Design review of the part built by this model. Coordinates are the model's own, in mm. Give positions to 0.01 mm unless a question says otherwise; leave off trailing zeros. Order: outer loops, then holes, each group sorted by start corner. A loop starts at its lowest first (then second) coordinate and runs counter-clockwise, first axis right, second up.
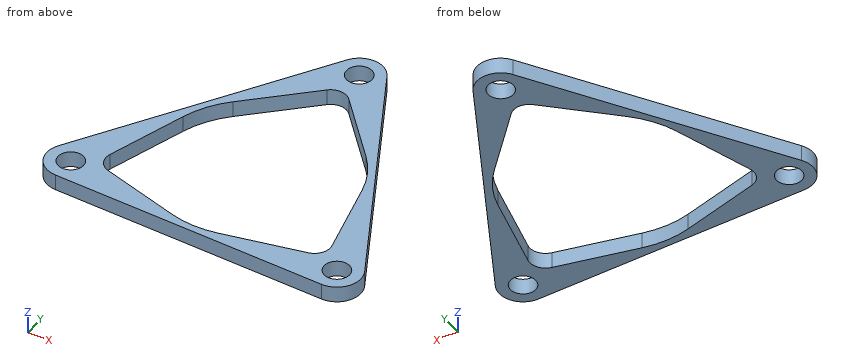
```python
from build123d import *

# Parameters (mm, degrees)
SKETCH1_R           = 3
SKETCH1_R_2         = 1.6
BOSS_EXTRUDE1_DEPTH = 2


with BuildPart() as part:
    # Sketch1 → Boss-Extrude1 (new body)
    # profile 1 of 4: a face of its own
    with BuildSketch(Plane.XY):
        with BuildLine():
            ThreePointArc((3.814909487, 19.983391167), (-0.020434351, 17.102037202), (-1.719890963, 21.588005352))
            Line((-1.719890963, 21.588005352), (-20.248379597, -7.681349081))
            ThreePointArc((-20.248379597, -7.681349081), (-16.87823531, -6.404609301), (-14.713579148, -9.285963266))
            ThreePointArc((-14.713579148, -9.285963266), (-15.635925335, -11.450069233), (-17.835815571, -12.283471941))
            Line((-17.835815571, -12.283471941), (16.776433238, -13.694936576))
            ThreePointArc((16.776433238, -13.694936576), (14.363869212, -9.092813716), (19.555706533, -9.304533411))
            Line((19.555706533, -9.304533411), (3.471946359, 21.376285657))
            ThreePointArc((3.471946359, 21.376285657), (3.727907136, 20.700639166), (3.814909487, 19.983391167))
        make_face()
        with BuildLine():
            Line((-8.306162696, 8.798730663), (-0.783837106, 15.899943621))
            ThreePointArc((-0.783837106, 15.899943621), (0.670573296, 16.443947091), (2.075859948, 15.783327064))
            Line((2.075859948, 15.783327064), (8.995004486, 8.093200498))
            ThreePointArc((8.995004486, 8.093200498), (10.716715384, 5.618007776), (11.773005623, 2.793982571))
            Line((11.773005623, 2.793982571), (14.161673647, -7.271148964))
            ThreePointArc((14.161673647, -7.271148964), (13.905589271, -8.802707055), (12.63083222, -9.689410982))
            Line((12.63083222, -9.689410982), (2.511414986, -11.836502641))
            ThreePointArc((2.511414986, -11.836502641), (-0.493020239, -12.089951656), (-3.466842927, -11.592713234))
            Line((-3.466842927, -11.592713234), (-13.377836541, -8.628794657))
            ThreePointArc((-13.377836541, -8.628794657), (-14.576162567, -7.641240036), (-14.706692168, -6.093916082))
            Line((-14.706692168, -6.093916082), (-11.506419472, 3.743302143))
            ThreePointArc((-11.506419472, 3.743302143), (-10.223695145, 6.47194388), (-8.306162696, 8.798730663))
        make_face(mode=Mode.SUBTRACT)
    # profile 2 of 4: a face of its own
    with BuildSketch(Plane.XY):
        with Locations((0.814909487, 19.983391167)):
            Circle(SKETCH1_R)
        with Locations((0.814909487, 19.983391167)):
            Circle(SKETCH1_R_2, mode=Mode.SUBTRACT)
    # profile 3 of 4: a face of its own
    with BuildSketch(Plane.XY):
        with Locations((16.898669661, -10.697427901)):
            Circle(SKETCH1_R)
        with Locations((16.898669661, -10.697427901)):
            Circle(SKETCH1_R_2, mode=Mode.SUBTRACT)
    # profile 4 of 4: a face of its own
    with BuildSketch(Plane.XY):
        with Locations((-17.713579148, -9.285963266)):
            Circle(SKETCH1_R)
        with Locations((-17.713579148, -9.285963266)):
            Circle(SKETCH1_R_2, mode=Mode.SUBTRACT)
    extrude(amount=BOSS_EXTRUDE1_DEPTH)


solid = part.part
```
1. Take a section at C-C (z = 1.1). State the section outline as (x, y) points (1 decimal), then the cut area to 3 significant figures.
Recorded:
outline: (-20.2, -7.7) arc R3 ccw to (-17.8, -12.3) - (16.8, -13.7) arc R3 ccw to (19.6, -9.3) - (3.5, 21.4) arc R3 ccw to (-1.7, 21.6) - close; hole circle Ø3.2 at (-17.7, -9.3); hole (-14.7, -6.1) arc R2 ccw to (-13.4, -8.6) - (-3.5, -11.6) arc R12.1 ccw to (2.5, -11.8) - (12.6, -9.7) arc R2 ccw to (14.2, -7.3) - (11.8, 2.8) arc R12.1 ccw to (9, 8.1) - (2.1, 15.8) arc R2 ccw to (-0.8, 15.9) - (-8.3, 8.8) arc R12.1 ccw to (-11.5, 3.7) - close; hole circle Ø3.2 at (0.8, 20); hole circle Ø3.2 at (16.9, -10.7)
area: 279 mm2
2. For pin 1 (1 mm diameter, centred on x = -3, z = 0.5, fed in from -Y), flat-tipped, find the tip position at first contact; note if it passes through.
Recorded:
pin 1: stops at y = -12.91
3. Take a section at D-D (y = 17). State the section outline as (x, z) points.
Recorded:
outline: (-4.62, 0) - (5.77, 0) - (5.77, 2) - (-4.62, 2) - close
4. For line 1 along Y through (x, z) = (-0.5, 1.75) (3 decimals); line 2 along Y through (x, z) = (1.5, 1.7); line 3 along Y through (x, z) = (-4, 0.7), list the stretches that pass through material, from the lowest coordinate up.
Recorded:
line 1: y = -12.99 to -12.09, 16.123 to 19.072, 20.895 to 22.68
line 2: y = -13.07 to -12.01, 16.23 to 18.54, 21.43 to 22.9
line 3: y = -12.85 to -11.43, 12.86 to 17.99
5. Take a section at A-A (x = 8). State the section outline as (y, z) points, then the cut area to 3 significant figures.
Recorded:
outline: (-13.34, 0) - (-10.67, 0) - (-10.67, 2) - (-13.34, 2) - close; (9.2, 0) - (12.74, 0) - (12.74, 2) - (9.2, 2) - close
area: 12.4 mm2
6. Take a section at B-B (y = 10). State the section outline as (x, z) points.
Recorded:
outline: (-9.06, 0) - (-7.03, 0) - (-7.03, 2) - (-9.06, 2) - close; (7.28, 0) - (9.44, 0) - (9.44, 2) - (7.28, 2) - close
